Autodesk Inventor part; units mm, degrees
ref_plane "YZ Plane" through (0, 0, 0) normal (1, 0, 0) x (0, 1, 0)
ref_plane "XZ Plane" through (0, 0, 0) normal (0, 1, 0) x (-1, 0, 0)
ref_plane "XY Plane" through (0, 0, 0) normal (0, 0, 1) x (1, 0, 0)
sketch "スケッチ1" plane through (0, 0, 0) normal (0, 0, 1) x (1, 0, 0)
  line L0 (-10.3125, 15) -> (-10.3125, -15)
  line L1 (-10.3125, -15) -> (0, -9.5)
  line L2 (0, -9.5) -> (0, 9.5)
  line L3 (0, 9.5) -> (-10.3125, 15)
  circle A0 centre (-2.5, 8) radius 1.55
  circle A1 centre (-2.5, -8) radius 1.55
  circle A2 centre (-2.5, 8) radius 2.5 construction
  circle A3 centre (-2.5, -8) radius 2.5 construction
  line L4 (-2.5, 8) -> (-2.5, -8) construction
  line L5 (-10.3125, 15) -> (59.873, -11.1505)
  line L6 (-10.3125, -15) -> (54.0766, -30.2519)
  arc A4 (54.0766, -30.2519) -> (59.873, -11.1505) centre (56.3816, -20.5212) ccw
  line L7 (56.3816, -20.5212) -> (0, 0) construction
  point P0 (-2.5, 0)
  dimension "d5" = 19
  dimension "d8" = 30
  dimension "d10" = 5
  dimension "d20" = 16
  dimension "d33" = 3.1
  dimension "d35" = 10
  dimension "d41" = 70
  dimension "d43" = 60
extrude "押し出し1" add sketch "スケッチ1" along normal blind 5
sketch "スケッチ4" plane through (0, 0, 0) normal (0, 0, -1) x (-1, 0, 0)
  circle A0 centre (2.5, 8) radius 1.55
  line L0 (-59.873, -11.1505) -> (10.3125, 15)
  arc A1 (-59.873, -11.1505) -> (-54.0766, -30.2519) centre (-56.3816, -20.5212) ccw
  line L1 (10.3125, -15) -> (-54.0766, -30.2519)
  line L2 (-2.5, -13.9242) -> (-54.9986, -26.3597)
  arc A2 (-58.4764, -14.8988) -> (-54.9986, -26.3597) centre (-56.3816, -20.5212) ccw
  line L3 (-58.4764, -14.8988) -> (-2.5, 5.9575)
  line L4 (-2.5, -13.9242) -> (-2.5, 5.9575)
  point P0 (0, 0)
  dimension "d81" = 4
  dimension "d82" = 5
extrude "押し出し4" cut sketch "スケッチ4" against normal blind 4 contours L2 A2 L3 L4
fillet "フィレット4" radius 2 2 edges at (2.5, 5.9575, 2) (2.5, -13.9242, 2)
equation "\"d5\" = d187"
equation "\"d8\" = d98"
equation "\"d10\" = d185"
equation "\"d20\" = d186"
equation "\"d185\" = 5"
equation "\"d187\" = 19"
properties part number "胴体_サブフレーム_1_6" material "アセタール樹脂、黒"
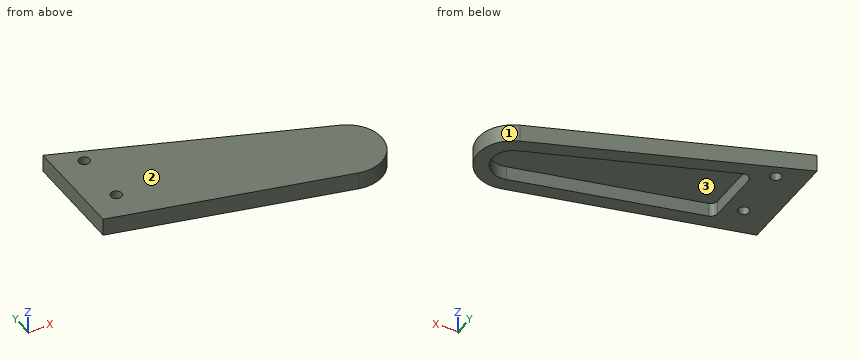
Geometry: final body of the model. Coordinates: model frame, mm. Face numbers are marked on the shaded views. Give positions to 0.01 mm unless a question says otherwise; leave off trailing zeros. Order: outer loops, then holes, each group sorted by start corner. A loop starts at its lowest first (then second) coordinate and runs counter-clockwise, first axis right, second up. Notation, with made-up numbers: (-29.75, -30) -> (9.25, -30) arc R15 cw to (9.25, -8) -> close; hole circle Ø2 at (68, 20.25). An arc over 180 degrees is marked (long way). Write each question's results on one line, items separated by ' | '.
1) Cut plane B-B (z = 1.3). Output: boundary loops of the cut face in (x, y).
Geometry says:
outline: (-10.31, -15) -> (54.08, -30.25) arc R10 ccw to (59.87, -11.15) -> (-10.31, 15) -> close; hole circle Ø3.1 at (-2.5, -8); hole circle Ø3.1 at (-2.5, 8); hole (2.5, -12.34) arc R2 ccw to (4.04, -14.29) -> (55, -26.36) arc R6 ccw to (58.48, -14.9) -> (5.2, 4.95) arc R2 ccw to (2.5, 3.08) -> close
2) First-contact query: pin 1 Ø1 at (x, z) = (9.5, 4) entering from -Y; pin 2 Ø5 at (x, y) = (-2.5, 8) entering from -Z; pin 3 Ø3 at (x, z) = (6.5, 1) entering from +Y. Flat tips, straight axial feed; report the tip coordinate or a pass-through.
Geometry says:
pin 1: stops at y = -19.81 | pin 2: stops at z = 0 | pin 3: stops at y = 9.29
3) Cut plane A-A (y = 8). Output: boundary loops of the cut face in (x, z), and give its area (3 significant figures).
Geometry says:
outline: (-10.31, 0) -> (-4.05, 0) -> (-4.05, 5) -> (-10.31, 5) -> close; (-0.95, 0) -> (8.47, 0) -> (8.47, 5) -> (-0.95, 5) -> close | area: 78.4 mm²
4) Line query: line 1 along Y through (x, z) = (-2.5, 1.85); line 2 along Z through (x, y) = (38, -9); line 3 along Y through (x, z) = (32, 0.75). Output: solid intervals per line, ascending.
Geometry says:
line 1: y = -16.85 to -9.55, -6.45 to 6.45, 9.55 to 12.09 | line 2: z = 4 to 5 | line 3: y = -25.02 to -20.91, -5.03 to -0.77
5) Cut plane D-D (x = 36.5). Output: boundary loops of the cut face in (y, z), and give its area (3 significant figures).
Geometry says:
outline: (-26.09, 0) -> (-21.98, 0) -> (-21.98, 4) -> (-6.71, 4) -> (-6.71, 0) -> (-2.44, 0) -> (-2.44, 5) -> (-26.09, 5) -> close | area: 57.2 mm²
6) Cut plane C-C (x = -3). Output: boundary loops of the cut face in (y, z).
Geometry says:
outline: (-16.73, 0) -> (-9.47, 0) -> (-9.47, 5) -> (-16.73, 5) -> close; (-6.53, 0) -> (6.53, 0) -> (6.53, 5) -> (-6.53, 5) -> close; (9.47, 0) -> (12.28, 0) -> (12.28, 5) -> (9.47, 5) -> close
7) Draft query along Y for the marked faces 1, 2 and 3. Return one class per face: released by +Y, released by -Y, zero draft, split by the parting line, or undercut.
Geometry says:
face 1: split by the parting line | face 2: zero draft | face 3: undercut
